from build123d import *

# Parameters (mm, degrees)
F0_W     = 5.08
F0_H     = 44.449404
F1_DEPTH = 149.86
F2_DEPTH = 1.5875
F3_W     = 7.62
F3_H     = 6.35
F3_W_2   = 50.8
F4_DEPTH = 1.778
F5_R     = 16.3195
F6_DEPTH = 6.096


with BuildPart() as f1:
    # F0 (on Front) → F1 (new body)
    with BuildSketch(Plane.XZ):
        with Locations((-2.54, 22.224702)):
            Rectangle(F0_W, F0_H)
    extrude(amount=F1_DEPTH)

    # F0 (on Front) → F2 (join)
    with BuildSketch(Plane.XZ):
        Polygon((-14.732, 0), (-5.08, 0), (-5.08, 44.449404), (0, 44.449404), (0, 68.834), (-14.732, 68.834), align=None)
    extrude(amount=F2_DEPTH)

    # F3 (on face) → F4 (join)
    with BuildSketch(Plane.YZ):
        with Locations((-74.93, -3.175)):
            Rectangle(F3_W, F3_H)
        with Locations((-106.68, -3.175)):
            Rectangle(F3_W_2, F3_H)
    extrude(amount=-F4_DEPTH)

    # F5 (on face) → F6 (join)
    with BuildSketch(Plane(origin=(-5.08, 0, 0), x_dir=(0, -1, 0), z_dir=(-1, 0, 0))):
        with Locations((115.7605, 22.224702)):
            Circle(F5_R)
    extrude(amount=F6_DEPTH)


solid = f1.part
Input: part model. Units: mm. Frame: model coordinates. A direction names the side the tool comes from. Give positions to 0.01 mm unless a question says otherwise; leave off trailing zeros. Write each loop counter-clockwise with the first axis right and the second up, starting at its lowest first coordinate (ties: lowest second). Pieces come first, ordered by that corner, then holes.
Q1. Section A-A, the plane x = -9.25. Output: boundary loops of the cut face in (y, z), plus the area to 3 significant figures.
Q2. First-contact query: P1, Ø1, axis at y = -106, z = 28.5, coming from the -X side; P2, Ø13.5, axis at y = -41.5, z = 17, coming from the -X side; P3, Ø8, axis at y = -20.5, z = 23.5, coming from the +X side; P4, Ø2, axis at x = -9.5, y = -104, coming from the +Z side. Flat tips, straight axial feed; report the tip coordinate or a pass-through.
Q3. Section D-D, the plane y = -134.5. Output: boundary loops of the cut face in (x, z), plus the area to 3 significant figures.
Q4. Section C-C, the plane y = -93.5. Output: boundary loops of the cut face in (x, z), plus the area to 3 significant figures.
Q5. Section B-B, the plane z = 12.5. Output: boundary loops of the cut face in (x, y), plus the area to 3 significant figures.
Q6. Material intervals for probe 1 along X at (y, z) = (-47, 42); probe 2 along Y at (x, z) = (-10.75, 35); probe 3 along Y at (x, z) = (-9, 52.5), sorted ascending.
Q7. Pull-direction query (Y, two-part tool) for faces 1 (the face through (-7, 0, 35)), 2 (the face through (-11.176, -116, 22)), 3 (the face through (-8.085, -99.457, 22.942)); classes: pulls with the +Y half, pulls with the -Y half, needs draft (parallel to the pull), parting line crosses it, or undercut.
Q8. Set-up query: faces 4 (the face through (-3, -149.86, 23)), 5 (the face through (-9, -1.588, 35)), 6 (the face through (0, -74, 22)), 7 (the face through (-3, -75, 44.449)), 8 (the face through (-1.778, -75, -3)). Return all of +Z, -Z, +X, -X, +Y, -Y with unobstructed straight access to the full face (end or side cutting, diameter ignored); none if empty.
Filled in:
1. outline: circle Ø32.64 at (-115.76, 22.22); (-1.59, 0) - (0, 0) - (0, 68.83) - (-1.59, 68.83) - close
1. area: 946 mm2
2. P1: stops at x = -11.18
2. P2: stops at x = -5.08
2. P3: stops at x = 0
2. P4: stops at z = 34.49
3. outline: (-5.08, 0) - (0, 0) - (0, 44.45) - (-5.08, 44.45) - close
3. area: 226 mm2
4. outline: (-5.08, 0) - (-1.78, 0) - (-1.78, -6.35) - (0, -6.35) - (0, 44.45) - (-5.08, 44.45) - close
4. area: 237 mm2
5. outline: (-14.73, -1.59) - (-5.08, -1.59) - (-5.08, -102.65) - (-11.18, -102.65) - (-11.18, -128.87) - (-5.08, -128.87) - (-5.08, -149.86) - (0, -149.86) - (0, 0) - (-14.73, 0) - close
5. area: 936 mm2
6. probe 1: x = -5.08 to 0
6. probe 2: y = -125.92 to -105.61, -1.59 to 0
6. probe 3: y = -1.59 to 0
7. face 1: pulls with the +Y half
7. face 2: needs draft
7. face 3: undercut
8. face 4: +Z, -Z, +X, -X, -Y
8. face 5: +Z, -X
8. face 6: +Z, -Z, +X, +Y, -Y
8. face 7: +Z, +X, -X, -Y
8. face 8: -Z, -X, +Y, -Y
